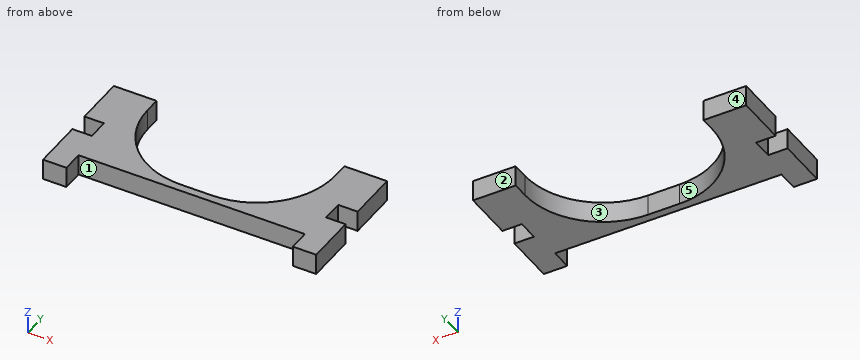
from build123d import *

# Parameters (mm, degrees)
BOSS_EXTRUDE1_DEPTH = 5.35


with BuildPart() as part:
    # Model → Boss-Extrude1 (new body)
    with BuildSketch(Plane.XY):
        with BuildLine():
            Line((-29, 0), (29, 0))
            Line((29, 0), (29, -5.35))
            Line((29, -5.35), (35, -5.35))
            Line((35, -5.35), (35, -2.50087083))
            Line((35, -2.50087083), (35, 7.65))
            Line((35, 7.65), (30, 7.65))
            Line((30, 7.65), (30, 13))
            Line((30, 13), (35, 13))
            Line((35, 13), (35, 26))
            Line((35, 26), (24.055, 26))
            Line((24.055, 26), (24.055, 22))
            ThreePointArc((24.055, 22), (18.197135624, 7.857864376), (4.055, 2))
            Line((4.055, 2), (-4.055, 2))
            ThreePointArc((-4.055, 2), (-18.197135624, 7.857864376), (-24.055, 22))
            Line((-24.055, 22), (-24.055, 26))
            Line((-24.055, 26), (-35, 26))
            Line((-35, 26), (-35, 13))
            Line((-35, 13), (-30, 13))
            Line((-30, 13), (-30, 7.65))
            Line((-30, 7.65), (-35, 7.65))
            Line((-35, 7.65), (-35, -2.50087083))
            Line((-35, -2.50087083), (-35, -5.35))
            Line((-35, -5.35), (-29, -5.35))
            Line((-29, -5.35), (-29, 0))
        make_face()
    extrude(amount=BOSS_EXTRUDE1_DEPTH)


solid = part.part
Verification items for the finished model (mm, model axes). Face numbers are marked on the shaded views. A direction names the side the tool comes from. Give positions to 0.01 mm unless a question says otherwise; leave off trailing zeros. Loops run counter-clockwise (first coordinate to the right, second up) from the corner with the lowest first, then second, coordinate; pieces in that order, holes last. Notation, with made-up numbers: (75.5, 61) - (98.5, 61) arc R13 cw to (98.5, 85) - close; hole circle Ø10 at (67, -6.5). An arc over 180 degrees is marked (long way). Write each question's results on one line, items separated by ' | '.
1) Tool access check on the marked faces 4 and 5. Record the directions out of +Z, -Z, +X, -X, +Y, -Y that give a thin tool (end or side, any length) a straight path to the whole face; none if there is none.
Solution:
face 4: +Z, -Z, +X, -X, +Y | face 5: +Z, -Z, +Y
2) Sectioned sample at D-D on y = 10.5. Record the boundary of the cut face in (x, z).
Solution:
outline: (-30, 0) - (-20.42, 0) - (-20.42, 5.35) - (-30, 5.35) - close; (20.42, 0) - (30, 0) - (30, 5.35) - (20.42, 5.35) - close
3) Sectioned sample at A-A on y = 24. Record the boundary of the cut face in (x, z) (3 decimals).
Solution:
outline: (-35, 0) - (-24.055, 0) - (-24.055, 5.35) - (-35, 5.35) - close; (24.055, 0) - (35, 0) - (35, 5.35) - (24.055, 5.35) - close
4) Material ranges on L1, parallel to X at y = -4, z = 2.6; L2, parallel to Y at x = 27, z = 3.3; L3, parallel to Y at x = -30.5, z = 1.75, recorded low to high. Write a range as from..to.
Solution:
L1: -35..-29, 29..35 | L2: 0..26 | L3: -5.35..7.65, 13..26
5) Mould release check, pull along X, two halves, no side actions. Record for the marked faces 1, 2 and 3: pulls with the +X half, pulls with the -X half, needs draft (parallel to the pull), parting line crosses it, or undercut.
Solution:
face 1: undercut | face 2: needs draft | face 3: undercut
6) Sectioned sample at C-C on x = -1. Record the boundary of the cut face in (y, z), plus the area to 3 significant figures.
Solution:
outline: (0, 0) - (2, 0) - (2, 5.35) - (0, 5.35) - close | area: 10.7 mm2
7) Depth check by flat-ended pin: P1, Ø3, axis at x = 5, z = 2.5, coming from the -Y side; P2, Ø1.6, axis at y = 9.5, z = 3.5, coming from the -X side; P3, Ø1, axis at y = 9, z = 2, coming from the +X side. Enter the tip coordinate at first touch or a pass-through.
Solution:
P1: y = 0 | P2: x = -30 | P3: x = 30
8) Sectioned sample at B-B on z = 1.75. Record the boundary of the cut face in (x, y) (3 decimals).
Solution:
outline: (-35, -5.35) - (-29, -5.35) - (-29, 0) - (29, 0) - (29, -5.35) - (35, -5.35) - (35, 7.65) - (30, 7.65) - (30, 13) - (35, 13) - (35, 26) - (24.055, 26) - (24.055, 22) arc R20 cw to (4.055, 2) - (-4.055, 2) arc R20 cw to (-24.055, 22) - (-24.055, 26) - (-35, 26) - (-35, 13) - (-30, 13) - (-30, 7.65) - (-35, 7.65) - close
